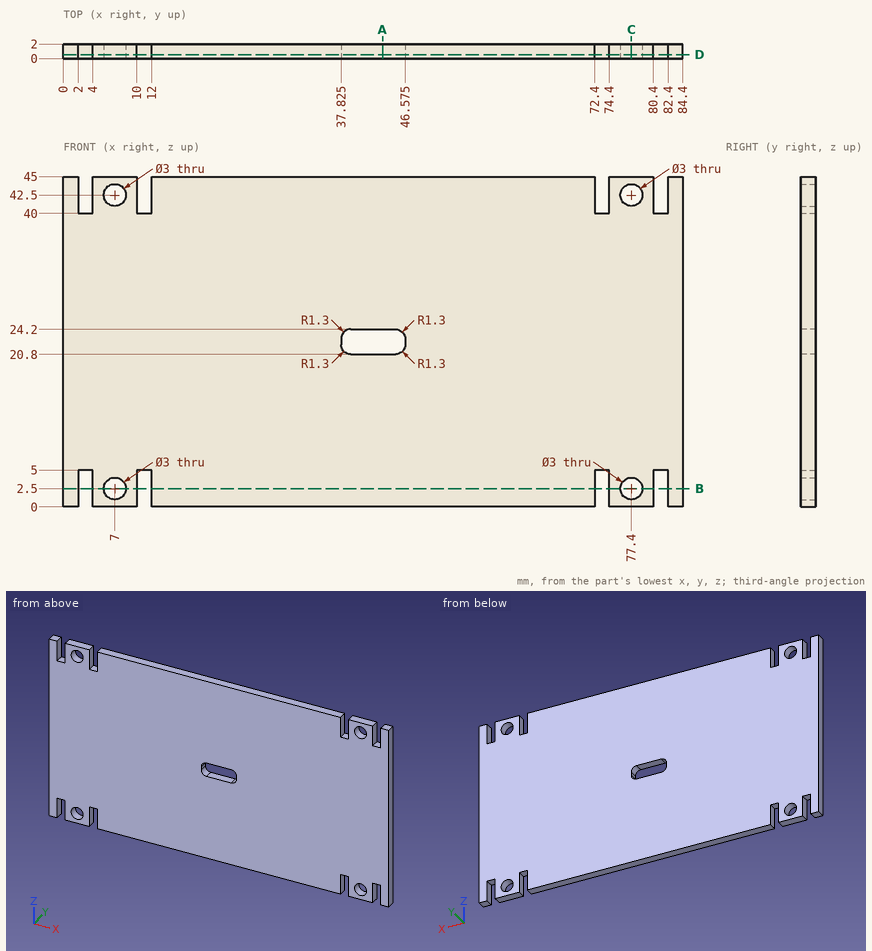
Here's the drawing with two shaded views (mm, measured from the low corner). I have some questions. Give positions to 0.01 mm unless a question says otherwise; leave off trailing zeros. Order: outer loops, then holes, each group sorted by start corner. A loop starts at its lowest first (then second) coordinate and runs counter-clockwise, first axis right, second up. Notation, with made-up numbers: (87.25, 42) - (124.25, 42) arc R16 ccw to (124.25, 72) - close; hole circle Ø1 at (59, 77.25). An arc over 180 degrees is marked (long way). Use a Markdown table: item, result. Add a question column.
Q1. If we section it at C-C on x = 77.4: Write out the boundary of the cut face in (y, z), plus the area to 3 significant figures.
Q2. If we section it at A-A on x = 43.5: Write out the boundary of the cut face in (y, z).
Q3. I'm going to push flat-ended pins straight in: pin 1 (0.6 mm diameter, centred on x = 73.5, y = 1, fed in from -Z); pin 2 (0.6 mm diameter, centred on x = 3.5, y = 0.5, fed in from +Z). Where does each tip first touch, or does it pass through?
Q4. If we section it at B-B on z = 2.5: Write out the boundary of the cut face in (x, y).
Q5. If we section it at D-D on y = 0.55: Count the separate pieces of the cut face and the enclosed holes in it, plus the area to 3 significant figures.
Q6. Please list where these lines run through material, in increasing order: line 1 along X through (y, z) = (1.45, 4.5); line 2 along Z through (x, y) = (77.5, 0.75); line 3 along Z through (x, y) = (44, 1.1).
Answers follow:
| question | item | result |
|---|---|---|
| 1 | outline | (0, 0) - (2, 0) - (2, 1) - (0, 1) - close; (0, 4) - (2, 4) - (2, 41) - (0, 41) - close; (0, 44) - (2, 44) - (2, 45) - (0, 45) - close |
| 1 | area | 78.0 mm^2 |
| 2 | outline | (0, 0) - (2, 0) - (2, 20.8) - (0, 20.8) - close; (0, 24.2) - (2, 24.2) - (2, 45) - (0, 45) - close |
| 3 | pin 1 | stops at z = 5 |
| 3 | pin 2 | stops at z = 40 |
| 4 | outline | (0, 0) - (2, 0) - (2, 2) - (0, 2) - close; (4, 0) - (5.5, 0) - (5.5, 2) - (4, 2) - close; (8.5, 0) - (10, 0) - (10, 2) - (8.5, 2) - close; (12, 0) - (72.4, 0) - (72.4, 2) - (12, 2) - close; (74.4, 0) - (75.9, 0) - (75.9, 2) - (74.4, 2) - close; (78.9, 0) - (80.4, 0) - (80.4, 2) - (78.9, 2) - close; (82.4, 0) - (84.4, 0) - (84.4, 2) - (82.4, 2) - close |
| 5 | separate pieces | 1 |
| 5 | enclosed holes | 5 |
| 5 | area | 3,660 mm^2 |
| 6 | line 1 | x = 0 to 2, 4 to 10, 12 to 72.4, 74.4 to 80.4, 82.4 to 84.4 |
| 6 | line 2 | z = 0 to 1, 4 to 41, 44 to 45 |
| 6 | line 3 | z = 0 to 20.8, 24.2 to 45 |
